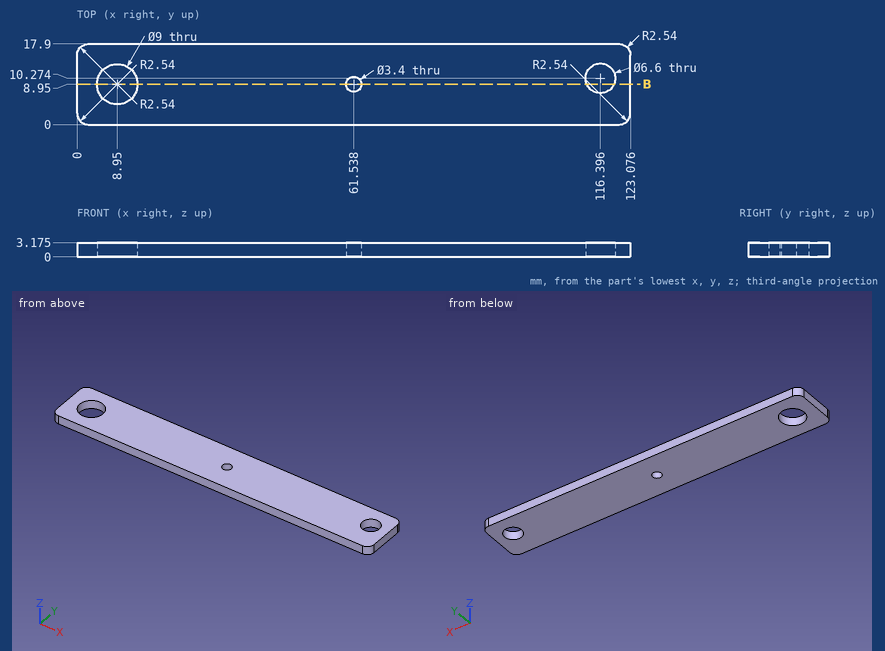
For this review, use the dimensioned drawing (mm, ordinates from the lowest corner) and the shaded views. Coordinates: 2 decimals unless noted, no trailing zeros. Return JSON: item names as keys, results as strings. Group by question number.
(1) To check wall thickness, follow L1, parallel to Y at x = 8.95, z = 1.2; L2, parallel to X at y = 12, z = 2.3 (1 decimal); L3, parallel to X at y = 11.25, z = 2.55 (1 decimal). State the ranges of each line that lie inside material, in increasing order.
(2) Consider section B-B, the plane y = 8.95. Count the separate pieces of the cut face and the enclosed holes in it, plus the area to 3 significant figures.
(3) For pin 1 Ø10.5 at (x, y) = (116.4, 10.27) entering from -Z, flat-tipped, find the tip position at first contact; note if it passes through.
Results below:
{
 "1": {"L1": "y = 0 to 4.45, 13.45 to 17.9", "L2": "x = 0 to 5.6, 12.3 to 113.6, 119.2 to 123.1", "L3": "x = 0 to 5.1, 12.8 to 113.2, 119.5 to 123.1"},
 "2": {"separate pieces": "4", "enclosed holes": "0", "area": "332 mm2"},
 "3": {"pin 1": "stops at z = 0"}
}
